Design review of the part built by this model. Coordinates are the model's own, in mm. A direction names the side the tool comes from. Coordinates: 2 decimals unless noted, no trailing zeros. Order: outer loops, then holes, each group sorted by start corner. A loop starts at its lowest first (then second) coordinate and runs counter-clockwise, first axis right, second up. Notation, with made-up numbers: M -15,-1.5 L 3,-1.5 A29 ccw 3,23.5 Z; hole C 30,19 d3. An arc over 180 degrees is marked long. Answer in a Markdown table with one row per item.
from build123d import *

# Parameters (mm, degrees)
SKETCH_2_R          = 7.5
EXTRUDE_2_DEPTH     = 21
SKETCH_3_R          = 3
EXTRUDE_3_DEPTH     = 2
SKETCH_4_R          = 1.5
EXTRUDE_4_DEPTH     = 6.9
CUT_EXTRUDE_START   = -6.5
CUT_EXTRUDE_1_DEPTH = 6.5
SKETCH_6_R          = 1
EXTRUDE_6_DEPTH     = 1.8
SKETCH_7_W          = 6
SKETCH_7_H          = 8
EXTRUDE_7_DEPTH     = 10


with BuildPart() as part:
    # 草图2 → 凸台-拉伸2 (new body)
    with BuildSketch(Plane.XY):
        with Locations(Location((0, 0, 0), (0, 0, 180))):
            Circle(SKETCH_2_R)
    extrude(amount=EXTRUDE_2_DEPTH)

    # 草图3 → 凸台-拉伸3 (add)
    with BuildSketch(Plane(origin=(0, 0, 0), x_dir=(-1, 0, 0), z_dir=(0, 0, -1))):
        Circle(SKETCH_3_R)
    extrude(amount=EXTRUDE_3_DEPTH)

    # 草图4 → 凸台-拉伸4 (add)
    with BuildSketch(Plane(origin=(0, 0, -2), x_dir=(-1, 0, 0), z_dir=(0, 0, -1))):
        with Locations(Location((0, 0, 0), (0, 0, 180))):
            Circle(SKETCH_4_R)
    extrude(amount=EXTRUDE_4_DEPTH)

    # 草图5 → 切除-拉伸1 (cut)
    with BuildSketch(Plane(origin=(0, 0, -8.9), x_dir=(-1, 0, 0), z_dir=(0, 0, -1)).offset(CUT_EXTRUDE_START)):
        with BuildLine():
            Line((-1.118033989, 1), (1.118033989, 1))
            ThreePointArc((1.118033989, 1), (0, 1.5), (-1.118033989, 1))
        make_face()
    extrude(amount=CUT_EXTRUDE_1_DEPTH, mode=Mode.SUBTRACT)

    # 草图6 → 凸台-拉伸6 (add)
    with BuildSketch(Plane(origin=(0, 0, 0), x_dir=(-1, 0, 0), z_dir=(0, 0, -1))):
        with BuildLine():
            Line((11.1, 1.670329309), (4.125, 6.263734908))
            ThreePointArc((4.125, 6.263734908), (0, 7.5), (-4.125, 6.263734908))
            Line((-4.125, 6.263734908), (-11.1, 1.670329309))
            ThreePointArc((-11.1, 1.670329309), (-12, 0), (-11.1, -1.670329309))
            Line((-11.1, -1.670329309), (-4.125, -6.263734908))
            ThreePointArc((-4.125, -6.263734908), (0, -7.5), (4.125, -6.263734908))
            Line((4.125, -6.263734908), (11.1, -1.670329309))
            ThreePointArc((11.1, -1.670329309), (12, 0), (11.1, 1.670329309))
        make_face()
        with Locations((10, 0)):
            Circle(SKETCH_6_R, mode=Mode.SUBTRACT)
        with Locations(Location((-10, 0, 0), (0, 0, 180))):
            Circle(SKETCH_6_R, mode=Mode.SUBTRACT)
    extrude(amount=-EXTRUDE_6_DEPTH)

    # 草图7 → 凸台-拉伸7 (add)
    with BuildSketch(Plane(origin=(0, 0, 0), x_dir=(0, 0, -1), z_dir=(1, 0, 0))):
        with Locations((-18, 0)):
            Rectangle(SKETCH_7_W, SKETCH_7_H)
    extrude(amount=EXTRUDE_7_DEPTH)


solid = part.part
(1) Insertion check: pin 1 Ø3 at (y, z) = (-1, 19) entering from +X; pin 2 Ø4.5 at (x, y) = (-4.5, 2.5) entering from -Z; pin 3 Ø2.5 at (x, y) = (-10, 0) entering from +Z. Each pin has a flat end and moves straight along its axis. Give the tip position at first contact, or say it passes through.
Return value:
| item | result |
|---|---|
| pin 1 | stops at x = 10 |
| pin 2 | stops at z = -2 |
| pin 3 | stops at z = 1.8 |
(2) Add section C-C, the plane x = 0. Give the boundary of the cut face in (y, z).
Return value:
| item | result |
|---|---|
| outline | M -7.5,0 L -3,0 L -3,-2 L -1.5,-2 L -1.5,-8.9 L 1,-8.9 L 1,-2.4 L 1.5,-2.4 L 1.5,-2 L 3,-2 L 3,0 L 7.5,0 L 7.5,21 L -7.5,21 Z |
(3) For faces 4 (the flat face through (10, 0, 18)), 5 (the flat face through (8, 4, 18)), 6 (the flat face through (7.661, -3.935, 0.887)), 7 (the flat face through (0, 1, -6)), 8 (the cylindrical face through (3, 0, -1)), list the 3-axis set-ups (+Z, -Z, +X, -X, +Y, -Y) from which the entire face can be reached by the end or side of a thin tool; tool diameter is ignored.
Return value:
| item | result |
|---|---|
| face 4 | +Z, +X, +Y, -Y |
| face 5 | +Z, +X, +Y |
| face 6 | -Z, +X, -Y |
| face 7 | -Z, +X, -X, +Y |
| face 8 | -Z |
(4) Add section D-D, the plane x = -10. Give the boundary of the cut face in (y, z).
Return value:
| item | result |
|---|---|
| outline | M -2.39,0 L -1,0 L -1,1.8 L -2.39,1.8 Z; M 1,0 L 2.39,0 L 2.39,1.8 L 1,1.8 Z |
(5) Add section A-A, the plane z = 0.5. Give the boundary of the cut face in (x, y) (3 decimals), and give its area (3 significant figures).
Return value:
| item | result |
|---|---|
| outline | M -11.1,-1.67 L -4.125,-6.264 A7.5 ccw 4.125,-6.264 L 11.1,-1.67 A2 ccw 11.1,1.67 L 4.125,6.264 A7.5 ccw -4.125,6.264 L -11.1,1.67 A2 ccw Z; hole C -10,0 d2; hole C 10,0 d2 |
| area | 226 mm2 |
(6) Draft analysis for pull direction Y (two halves, no side actions). For faces 1 (the cylindrical face through (12, 0, 1)), 2 (the cylindrical face through (9.2, 0.6, 0.9)), 3 (the flat face through (7.56, 4, 0.89)), state which applies: pulls with the +Y half, pulls with the -Y half, needs draft (parallel to the pull), parting line crosses it, or undercut.
Return value:
| item | result |
|---|---|
| face 1 | parting line crosses it |
| face 2 | undercut |
| face 3 | pulls with the +Y half |
(7) Add section B-B, the plane y = 0. Give the boundary of the cut face in (x, z), and give its area (3 significant figures).
Return value:
| item | result |
|---|---|
| outline | M -12,0 L -11,0 L -11,1.8 L -12,1.8 Z; M -9,0 L -3,0 L -3,-2 L -1.5,-2 L -1.5,-8.9 L 1.5,-8.9 L 1.5,-2 L 3,-2 L 3,0 L 9,0 L 9,1.8 L 7.5,1.8 L 7.5,15 L 10,15 L 10,21 L -7.5,21 L -7.5,1.8 L -9,1.8 Z; M 11,0 L 12,0 L 12,1.8 L 11,1.8 Z |
| area | 372 mm2 |
(8) For line 1 along Y through (x, z) = (10.25, 1.25); line 2 along Z through (x, y) = (3.5, -2.75); line 3 along Z through (x, y) = (-0.25, -2.5), list the stretches that pass through material, from the lowest coordinate up. Write a range as from..to.
Return value:
| item | result |
|---|---|
| line 1 | y = -2.23..-0.97, 0.97..2.23 |
| line 2 | z = 0..21 |
| line 3 | z = -2..21 |
